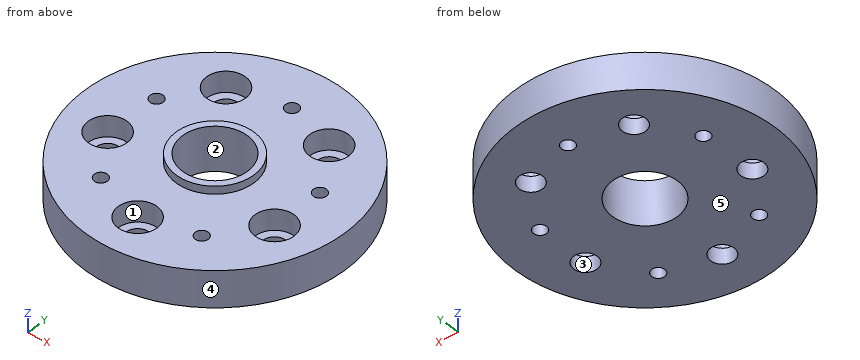
```python
from build123d import *

# Parameters (mm, degrees)
SKETCH1_R                      = 50
BOSS_EXTRUDE1_DEPTH            = 14
SKETCH2_R                      = 12.5
CUT_EXTRUDE1_DEPTH             = 73.083285164
BOSS_EXTRUDE2_START            = 3
SKETCH3_R                      = 15
SKETCH3_R_2                    = 12.5
BOSS_EXTRUDE2_DEPTH            = 3
CBORE_FOR_M8_SHCS1_D           = 9
CBORE_FOR_M8_SHCS1_CBORE_D     = 15
CBORE_FOR_M8_SHCS1_CBORE_DEPTH = 8
M6X1_0_TAPPED_HOLE1_D          = 5


with BuildPart() as part:
    # Sketch1 → Boss-Extrude1 (new body)
    with BuildSketch(Plane.XY):
        Circle(SKETCH1_R)
    extrude(amount=BOSS_EXTRUDE1_DEPTH)

    # Sketch2 → Cut-Extrude1 (cut, through all)
    with BuildSketch(Plane.XY.offset(14)):
        Circle(SKETCH2_R)
    extrude(amount=-CUT_EXTRUDE1_DEPTH, mode=Mode.SUBTRACT)

    # Sketch3 → Boss-Extrude2 (add)
    with BuildSketch(Plane.XY.offset(14).offset(BOSS_EXTRUDE2_START)):
        Circle(SKETCH3_R)
        Circle(SKETCH3_R_2, mode=Mode.SUBTRACT)
    extrude(amount=-BOSS_EXTRUDE2_DEPTH)

    # CBORE for M8 SHCS1 (through all)
    with Locations(Plane.XY.offset(14)):
        with Locations((0, -34), (-32.335921554, -10.506577809), (-19.984698578, 27.506577809), (19.984698578, 27.506577809), (32.335921554, -10.506577809)):
            CounterBoreHole(CBORE_FOR_M8_SHCS1_D / 2, CBORE_FOR_M8_SHCS1_CBORE_D / 2, CBORE_FOR_M8_SHCS1_CBORE_DEPTH)

    # M6x1.0 Tapped Hole1 (through all)
    with Locations(Plane.XY.offset(14)):
        with Locations((-19.984698578, -27.506577809), (-31.705846612, 10.30185405), (0.630074942, 33.132776241), (32.335921554, 9.434630291), (19.595290848, -28.042551568), (0.174148431, -0.535973759)):
            Hole(M6X1_0_TAPPED_HOLE1_D / 2)


solid = part.part
```
Design review of the part built by this model. Coordinates are the model's own, in mm. Face numbers are marked on the shaded views. A direction names the side the tool comes from. Coordinates: 2 decimals unless noted, no trailing zeros. Loops run counter-clockwise (first coordinate to the right, second up) from the corner with the lowest first, then second, coordinate; pieces in that order, holes last.
Q1. Tool access review of the marked faces 1 and 2: name each direction out of +Z, -Z, +X, -X, +Y, -Y from which nothing blocks a thin tool from reaching the whole face with its end or side.
Reported:
face 1: +Z
face 2: +Z, -Z
Q2. We need section C-C on x = 18.5. State the section outline as (y, z) points (3 decimals).
Reported:
outline: (-46.452, 0) - (-30.29, 0) - (-30.29, 14) - (-46.452, 14) - close; (-25.795, 0) - (23.259, 0) - (23.259, 6) - (20.155, 6) - (20.155, 14) - (-25.795, 14) - close; (31.755, 0) - (46.452, 0) - (46.452, 14) - (34.858, 14) - (34.858, 6) - (31.755, 6) - close
Q3. We need section B-B on x = 0. State the section outline as (y, z) points.
Reported:
outline: (-50, 0) - (-38.5, 0) - (-38.5, 6) - (-41.5, 6) - (-41.5, 14) - (-50, 14) - close; (-29.5, 0) - (-12.5, 0) - (-12.5, 17) - (-15, 17) - (-15, 14) - (-26.5, 14) - (-26.5, 6) - (-29.5, 6) - close; (12.5, 0) - (30.71, 0) - (30.71, 14) - (15, 14) - (15, 17) - (12.5, 17) - close; (35.55, 0) - (50, 0) - (50, 14) - (35.55, 14) - close
Q4. For pin 1 (8 mm diameter, centred on x = -32.34, y = -10.51, fed in from +Z); pin 2 (1 mm diameter, centred on x = 3.5, z = 8, fed in from +Y); pin 3 (4.5 mm diameter, centred on x = 35.5, y = -8.5, fed in from +Z); pin 4 (8 mm diameter, centred on x = -31.71, y = 10.3, fed in from +Z), all flat-tipped, find the tip position at first contact; note any pin that passes through.
Reported:
pin 1: passes through
pin 2: stops at y = 49.91
pin 3: stops at z = 6
pin 4: stops at z = 14
Q5. We need section D-D on y = -34. State the section outline as (x, z) points, and give its area (3 significant figures).
Reported:
outline: (-36.66, 0) - (-4.5, 0) - (-4.5, 6) - (-7.5, 6) - (-7.5, 14) - (-36.66, 14) - close; (4.5, 0) - (36.66, 0) - (36.66, 14) - (7.5, 14) - (7.5, 6) - (4.5, 6) - close
area: 852 mm2
Q6. The part is to be moulded in two halves that separate along X. For the marked faces 3, 4 and 5, say which applies: +X half, -X half, draft (parallel to the pull), parting line (faces both ways), or undercut.
Reported:
face 3: undercut
face 4: parting line
face 5: draft
Q7. To check wall thickness, follow line 1 (X direction, y = -13.5, z = 7.75); line 2 (X direction, y = 10.5, z = 7.75); line 3 (Y direction, x = 0, z = 11). State the ranges of each line that lie inside material, in increasing order.
Reported:
line 1: x = -48.14 to -39.21, -25.46 to 25.46, 39.21 to 48.14
line 2: x = -48.89 to -34.2, -29.21 to -6.78, 6.78 to 30.07, 34.6 to 48.89
line 3: y = -50 to -41.5, -26.5 to -12.5, 12.5 to 30.71, 35.55 to 50
Q8. We need section A-A on y = 0. State the section outline as (x, z) points.
Reported:
outline: (-50, 0) - (-12.5, 0) - (-12.5, 17) - (-15, 17) - (-15, 14) - (-50, 14) - close; (12.5, 0) - (50, 0) - (50, 14) - (15, 14) - (15, 17) - (12.5, 17) - close
